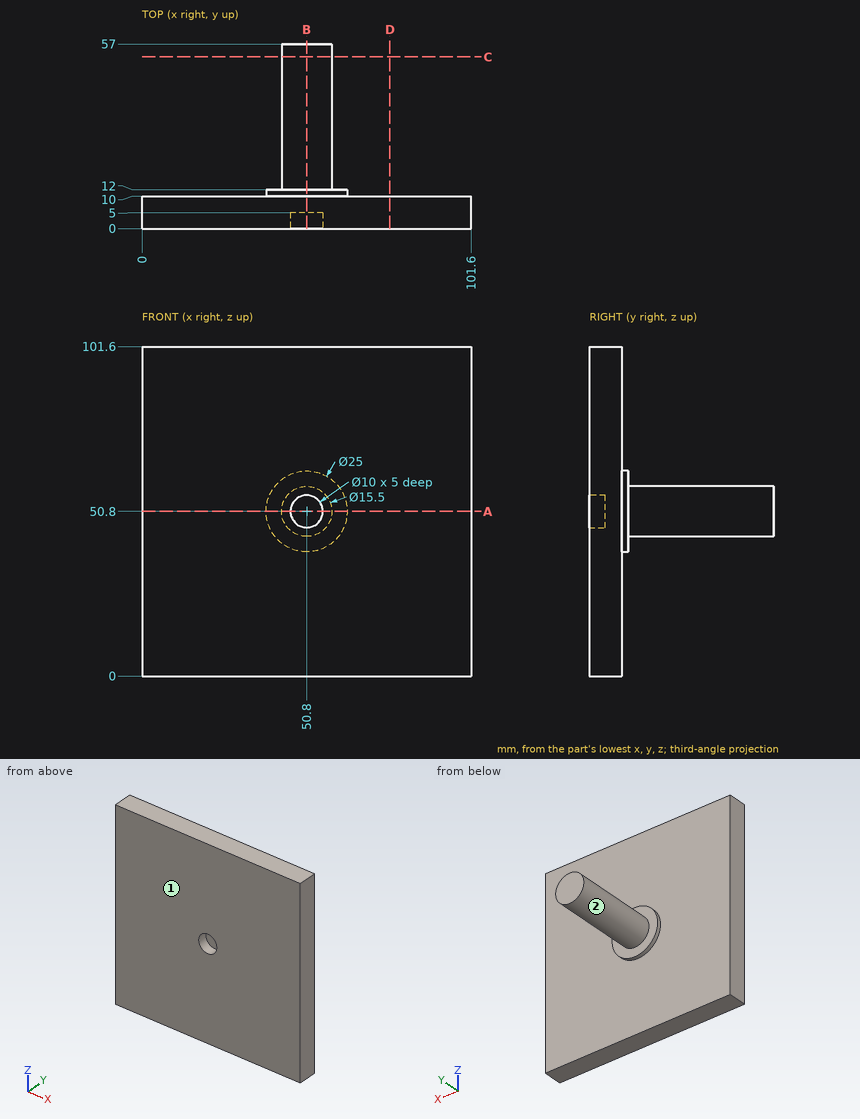
For this review, use the dimensioned drawing (mm, ordinates from the lowest corner) and the shaded views. A direction names the side the tool comes from. Coordinates: 2 decimals unless noted, no trailing zeros. Write each loop counter-clockwise with the first axis right and the second up, starting at its lowest first coordinate (ties: lowest second). Pieces come first, ordered by that corner, then holes. Notation, with made-up numbers: (49.5, 43.5) - (84.5, 43.5) arc R36 cw to (84.5, 78.5) - close; hole circle Ø9 at (12, 46.25). An arc over 180 degrees is marked (long way). Answer as a JSON object with one key per item and string values. Group by question number.
1. Add section A-A (z = 50.8). Give the boundary of the cut face in (x, y).
2. Add section C-C (y = 53). Give the boundary of the cut face in (x, z), plus the area to 3 significant figures.
3. Add section D-D (x = 76.5). Give the boundary of the cut face in (y, z), plus the area to 3 significant figures.
4. To check wall thickness, follow probe 1 along Y at (x, z) = (55.5, 95); probe 2 along Z at (x, y) = (50, 2); probe 3 along X at (y, z) = (1, 50.8). State the ranges of each line that lie inside material, in increasing order.
5. Clearance check with flat-ended pins moving along their axes: pin 1 Ø3 at (x, z) = (72.5, 38.5) entering from +Y; pin 2 Ø1 at (x, z) = (89.5, 39.5) entering from -Y. State where each tip first meets the part, or that it passes through.
6. Machinability: for the marked faces 1 and 2, which of the approach directions +Z, -Z, +X, -X, +Y, -Y give a long, thin tool a straight path to every point of the face, cutting with its end or side? Answer none if there is none.
7. Add section B-B (x = 50.8). Give the boundary of the cut face in (y, z), plus the area to 3 significant figures.
Findings:
{
 "1": {"outline": "(0, 0) - (45.8, 0) - (45.8, 5) - (55.8, 5) - (55.8, 0) - (101.6, 0) - (101.6, 10) - (63.3, 10) - (63.3, 12) - (58.55, 12) - (58.55, 57) - (43.05, 57) - (43.05, 12) - (38.3, 12) - (38.3, 10) - (0, 10) - close"},
 "2": {"outline": "circle Ø15.5 at (50.8, 50.8)", "area": "189 mm²"},
 "3": {"outline": "(0, 0) - (10, 0) - (10, 101.6) - (0, 101.6) - close", "area": "1,020 mm²"},
 "4": {"probe 1": "0 to 10", "probe 2": "0 to 45.86, 55.74 to 101.6", "probe 3": "0 to 45.8, 55.8 to 101.6"},
 "5": {"pin 1": "y = 10", "pin 2": "y = 0"},
 "6": {"face 1": "+Z, -Z, +X, -X, -Y", "face 2": "+Y"},
 "7": {"outline": "(0, 0) - (10, 0) - (10, 38.3) - (12, 38.3) - (12, 43.05) - (57, 43.05) - (57, 58.55) - (12, 58.55) - (12, 63.3) - (10, 63.3) - (10, 101.6) - (0, 101.6) - (0, 55.8) - (5, 55.8) - (5, 45.8) - (0, 45.8) - close", "area": "1,710 mm²"}
}
